Model file for the job. Use its own axes, mm. Round coordinates to 2 decimals unless told otherwise and drop trailing zeros. Write each loop counter-clockwise with the first axis right and the second up, starting at its lowest first coordinate (ties: lowest second). Pieces come first, ordered by that corner, then holes. Notation, with made-up numbers: (6.5, 62) - (22.5, 62) arc R25 ccw to (22.5, 88) - close; hole circle Ø8 at (84.5, 67). An arc over 180 degrees is marked (long way). Answer as a JSON object with one key per item and string values. Group by question number.
from build123d import *

# Parameters (mm, degrees)
SKETCH1_R           = 32.5
SKETCH1_R_2         = 24.095
SKETCH1_R_3         = 1.0625
BOSS_EXTRUDE1_DEPTH = 4.5
SCALE1_SCALE        = 25.4


with BuildPart() as part:
    # Sketch1 → Boss-Extrude1 (new body)
    with BuildSketch(Plane.XY):
        Circle(SKETCH1_R)
        Circle(SKETCH1_R_2, mode=Mode.SUBTRACT)
        with Locations((0, 30.375)):
            Circle(SKETCH1_R_3, mode=Mode.SUBTRACT)
        with Locations((4.751696876, 30.001033346)):
            Circle(SKETCH1_R_3, mode=Mode.SUBTRACT)
        with Locations((9.386391204, 28.888341682)):
            Circle(SKETCH1_R_3, mode=Mode.SUBTRACT)
        with Locations((13.78996143, 27.064323172)):
            Circle(SKETCH1_R_3, mode=Mode.SUBTRACT)
        with Locations((17.853977038, 24.573891204)):
            Circle(SKETCH1_R_3, mode=Mode.SUBTRACT)
        with Locations((21.478368479, 21.478368479)):
            Circle(SKETCH1_R_3, mode=Mode.SUBTRACT)
        with Locations((24.573891204, 17.853977038)):
            Circle(SKETCH1_R_3, mode=Mode.SUBTRACT)
        with Locations((27.064323172, 13.78996143)):
            Circle(SKETCH1_R_3, mode=Mode.SUBTRACT)
        with Locations((28.888341682, 9.386391204)):
            Circle(SKETCH1_R_3, mode=Mode.SUBTRACT)
        with Locations((30.001033346, 4.751696876)):
            Circle(SKETCH1_R_3, mode=Mode.SUBTRACT)
        with Locations((30.375, 0)):
            Circle(SKETCH1_R_3, mode=Mode.SUBTRACT)
        with Locations((30.001033346, -4.751696876)):
            Circle(SKETCH1_R_3, mode=Mode.SUBTRACT)
        with Locations((28.888341682, -9.386391204)):
            Circle(SKETCH1_R_3, mode=Mode.SUBTRACT)
        with Locations((27.064323172, -13.78996143)):
            Circle(SKETCH1_R_3, mode=Mode.SUBTRACT)
        with Locations((24.573891204, -17.853977038)):
            Circle(SKETCH1_R_3, mode=Mode.SUBTRACT)
        with Locations((21.478368479, -21.478368479)):
            Circle(SKETCH1_R_3, mode=Mode.SUBTRACT)
        with Locations((17.853977038, -24.573891204)):
            Circle(SKETCH1_R_3, mode=Mode.SUBTRACT)
        with Locations((13.78996143, -27.064323172)):
            Circle(SKETCH1_R_3, mode=Mode.SUBTRACT)
        with Locations((9.386391204, -28.888341682)):
            Circle(SKETCH1_R_3, mode=Mode.SUBTRACT)
        with Locations((4.751696876, -30.001033346)):
            Circle(SKETCH1_R_3, mode=Mode.SUBTRACT)
        with Locations((0, -30.375)):
            Circle(SKETCH1_R_3, mode=Mode.SUBTRACT)
        with Locations((-4.751696876, -30.001033346)):
            Circle(SKETCH1_R_3, mode=Mode.SUBTRACT)
        with Locations((-9.386391204, -28.888341682)):
            Circle(SKETCH1_R_3, mode=Mode.SUBTRACT)
        with Locations((-13.78996143, -27.064323172)):
            Circle(SKETCH1_R_3, mode=Mode.SUBTRACT)
        with Locations((-17.853977038, -24.573891204)):
            Circle(SKETCH1_R_3, mode=Mode.SUBTRACT)
        with Locations((-21.478368479, -21.478368479)):
            Circle(SKETCH1_R_3, mode=Mode.SUBTRACT)
        with Locations((-24.573891204, -17.853977038)):
            Circle(SKETCH1_R_3, mode=Mode.SUBTRACT)
        with Locations((-27.064323172, -13.78996143)):
            Circle(SKETCH1_R_3, mode=Mode.SUBTRACT)
        with Locations((-28.888341682, -9.386391204)):
            Circle(SKETCH1_R_3, mode=Mode.SUBTRACT)
        with Locations((-30.001033346, -4.751696876)):
            Circle(SKETCH1_R_3, mode=Mode.SUBTRACT)
        with Locations((-30.375, 0)):
            Circle(SKETCH1_R_3, mode=Mode.SUBTRACT)
        with Locations((-30.001033346, 4.751696876)):
            Circle(SKETCH1_R_3, mode=Mode.SUBTRACT)
        with Locations((-28.888341682, 9.386391204)):
            Circle(SKETCH1_R_3, mode=Mode.SUBTRACT)
        with Locations((-27.064323172, 13.78996143)):
            Circle(SKETCH1_R_3, mode=Mode.SUBTRACT)
        with Locations((-24.573891204, 17.853977038)):
            Circle(SKETCH1_R_3, mode=Mode.SUBTRACT)
        with Locations((-21.478368479, 21.478368479)):
            Circle(SKETCH1_R_3, mode=Mode.SUBTRACT)
        with Locations((-17.853977038, 24.573891204)):
            Circle(SKETCH1_R_3, mode=Mode.SUBTRACT)
        with Locations((-13.78996143, 27.064323172)):
            Circle(SKETCH1_R_3, mode=Mode.SUBTRACT)
        with Locations((-9.386391204, 28.888341682)):
            Circle(SKETCH1_R_3, mode=Mode.SUBTRACT)
        with Locations((-4.751696876, 30.001033346)):
            Circle(SKETCH1_R_3, mode=Mode.SUBTRACT)
    extrude(amount=BOSS_EXTRUDE1_DEPTH)


with BuildPart() as part_1:
    # Scale1: scaled about (0, 0, 2.25)
    add(part.part.scale(SCALE1_SCALE).moved(Location((0, 0, -54.9))))


solid = part_1.part
(1) Slice it at A-A (x = 0). Write the cut outline in (y, z), then the cut area to 3 significant figures.
(2) Flat gauge pins, fed straight in: pin 1 (1.5 mm diameter, centred on y = -641, z = -18, fed in from -X); pin 2 (1.5 mm diameter, centred on y = 283.5, z = 24.5, fed in from +X); pin 3 (1.5 mm diameter, centred on y = -119.5, z = -35.5, fed in from -X). Where does each tip first touch, or does it go through?
(3) Drill centre lines: line 1 (X direction, y = 332.5, z = -4.5); line 2 (X direction, y = 117, z = -26); line 3 (Y direction, x = -522.5, z = -27) (3 decimals). Where is each one in solid material? Low to high. Write a range as from..to.
(4) Pull direction X, two halves, no side cores. Call faces 1 (the cylindrical face through (-335.757, -664.678, 1.45)), 2 (the flat face through (-4, 615, -54.9)): pulls with the +X half, pulls with the -X half, needs draft (parallel to the pull), parting line crosses it, or undercut.
(5) Slice it at C-C (z = -2). Count the separate pieces of the cut face and the enclosed holes in it, then the cut area to 3 significant figures.
Answer:
{
 "1": {"outline": "(-825.5, -54.9) - (-798.51, -54.9) - (-798.51, 59.4) - (-825.5, 59.4) - close; (-744.54, -54.9) - (-612.01, -54.9) - (-612.01, 59.4) - (-744.54, 59.4) - close; (612.01, -54.9) - (744.54, -54.9) - (744.54, 59.4) - (612.01, 59.4) - close; (798.51, -54.9) - (825.5, -54.9) - (825.5, 59.4) - (798.51, 59.4) - close", "area": "36,500 mm²"},
 "2": {"pin 1": "x = -521.09", "pin 2": "x = 775.57", "pin 3": "x = -816.91"},
 "3": {"line 1": "-755.58..-707.75, -667.12..-513.81, 513.81..667.12, 707.75..755.58", "line 2": "-817.17..-788.76, -735.29..-600.73, 600.73..735.29, 788.76..817.17", "line 3": "-639.096..-559.586, -531.515..-318.675, 318.675..531.515, 559.586..639.096"},
 "4": {"face 1": "undercut", "face 2": "needs draft"},
 "5": {"separate pieces": "1", "enclosed holes": "41", "area": "873,000 mm²"}
}
